Autodesk Inventor part; units mm, degrees
ref_plane "Work Plane1" through (0, 0, 0) normal (0, 0, 1) x (1, 0, 0)
ref_plane "Work Plane2" through (0, 0, 4) normal (0, 0, -1) x (-1, 0, 0)
ref_plane "Work Plane3" through (-20.3, -49, 28.5) normal (0, -1, 0) x (1, 0, 0)
ref_plane "Work Plane1" through (0, 0, 0) normal (0, 0, 1) x (1, 0, 0)
sketch "Sketch1" plane through (0, 0, 0) normal (0, 0, 1) x (1, 0, 0)
  circle A0 centre (-17.3, 4) radius 1.35
  circle A1 centre (-17.3, -18) radius 1.35
  circle A2 centre (-17.3, -40) radius 1.35
  line L0 (-17.3, 4) -> (-14.8, 4)
  line L1 (-14.8, 4) -> (-14.8, 9)
  line L2 (-14.8, 9) -> (-20.3, 9)
  line L3 (-17.3, -40) -> (-17.3, -54)
  line L4 (-14.8, 4) -> (-14.8, -54)
  line L5 (-14.8, -54) -> (-17.3, -54)
  line L6 (-17.3, -54) -> (-20.3, -54)
  line L7 (-20.3, -54) -> (-20.3, 9)
  point P0 (0, 0)
  dimension "d0" = 2.5
  dimension "d1" = 5
  dimension "d2" = 5.5
  dimension "d3" = 14
extrude "Extrusion1" add sketch "Sketch1" along normal blind 36.5
sketch "Sketch2" plane through (-20.3, -54, 0) normal (0, -1, 0) x (1, 0, 0)
  line L0 (0, 0) -> (5.5, 0)
  line L1 (5.5, 0) -> (5.5, 36.5)
  line L2 (0, 36.5) -> (5.5, 36.5)
  line L3 (0, 0) -> (0, 36.5)
  line L4 (2.75, 36.5) -> (2.75, 25.5)
  circle A0 centre (2.75, 25.5) radius 1.5
  point P0 (20.3, 0)
  dimension "d6" = 11
  dimension "d7" = 3
extrude "Extrusion2" cut sketch "Sketch2" against normal blind 10 contours A0
sketch "Sketch3" plane through (-20.3, -54, 0) normal (-1, 0, 0) x (0, 0, 1)
  line L0 (0, 63) -> (0, 0)
  line L1 (0, 0) -> (36.5, 0)
  line L2 (36.5, 63) -> (36.5, 0)
  line L3 (0, 63) -> (36.5, 63)
  line L4 (0, 0) -> (36.5, 0)
  line L5 (36.5, 0) -> (28.5, 0)
  line L6 (28.5, 0) -> (28.5, 8)
  line L7 (28.5, 8) -> (36.5, 8)
  line L8 (36.5, 8) -> (36.5, 0)
  point P0 (0, 54)
  dimension "d10" = 8
  dimension "d11" = 8
extrude "Extrusion3" cut sketch "Sketch3" against normal blind 10 contours L6 L7 L2 L1
sketch "Sketch4" plane through (-20.3, 9, 0) normal (0, 1, 0) x (1, 0, 0)
  line L0 (5.5, 0) -> (0, 0)
  line L1 (0, 0) -> (0, -36.5)
  line L2 (5.5, -36.5) -> (0, -36.5)
  line L3 (5.5, 0) -> (5.5, -36.5)
  line L4 (6.8, -6) -> (8.8, -6)
  line L5 (6.8, -6) -> (5.5, -6)
  line L6 (5.5, -6) -> (5.5, -6.5)
  line L7 (5.5, 0) -> (5.5, -28.5)
  line L8 (5.5, -6.5) -> (15.5, -6.5)
  line L9 (15.5, -6.5) -> (15.5, -11.5)
  line L10 (15.5, -11.5) -> (5.5, -11.5)
  line L11 (5.5, -11.5) -> (5.5, -6.5)
  point P0 (20.3, 0)
  dimension "d14" = 0.5
  dimension "d15" = 10
  dimension "d16" = 5
extrude "Extrusion4" add sketch "Sketch4" against normal up to surface (63 mm away) contours L8 L9 L10 L3
sketch "Sketch5" plane through (-4.8, 9, 6.5) normal (0, 0, -1) x (-1, 0, 0)
  circle A0 centre (12.5, -49) radius 1.35
  circle A1 centre (12.5, -27) radius 1.35
  circle A2 centre (12.5, -5) radius 1.35
  line L0 (10, -63) -> (10, 0)
  line L1 (15.5, -63) -> (10, -63)
  line L2 (15.5, 0) -> (15.5, -63)
  line L3 (10, 0) -> (15.5, 0)
  line L4 (0, -63) -> (10, -63)
  line L5 (10, 0) -> (10, -63)
  line L6 (0, 0) -> (10, 0)
  line L7 (0, 0) -> (0, -63)
  line L8 (-19.8, 5.5) -> (-16.3, 5.5)
  line L9 (-19.8, 5.5) -> (-24.9, -0.5)
  line L10 (-24.9, -0.5) -> (-24.9, -53.6)
  line L11 (-24.9, -53.6) -> (-19.8, -59.6)
  line L12 (-19.8, -59.6) -> (10.2, -59.6)
  line L13 (10.2, -59.6) -> (15.3, -53.6)
  line L14 (15.3, -53.6) -> (15.3, -0.5)
  line L15 (15.3, -0.5) -> (10.2, 5.5)
  line L16 (6.7, 5.5) -> (10.2, 5.5)
  arc A3 (9.7, 2.5) -> (6.7, 5.5) centre (6.7, 2.5) ccw
  line L17 (9.7, -51) -> (9.7, 2.5)
  arc A4 (6.7, -54) -> (9.7, -51) centre (6.7, -51) ccw
  line L18 (-16.3, -54) -> (6.7, -54)
  arc A5 (-19.3, -51) -> (-16.3, -54) centre (-16.3, -51) ccw
  line L19 (-19.3, 2.5) -> (-19.3, -51)
  arc A6 (-16.3, 5.5) -> (-19.3, 2.5) centre (-16.3, 2.5) ccw
  circle A7 centre (12.5, -5) radius 1.35
  circle A8 centre (12.5, -27) radius 1.35
  circle A9 centre (12.5, -49) radius 1.35
  circle A10 centre (6.2, -56.8) radius 1.35
  circle A11 centre (-22.1, -5) radius 1.35
  circle A12 centre (-22.1, -27) radius 1.35
  circle A13 centre (-22.1, -49) radius 1.35
  circle A14 centre (-15.8, -56.8) radius 1.35
  line L20 (10, 0) -> (10, -63)
  line L21 (10, -63) -> (0, -63)
  line L22 (0, -63) -> (0, -54.5)
  line L23 (0, -54.5) -> (10, -54.5)
  line L24 (10, -54.5) -> (10, -63)
  point P0 (-4.8, -9)
  dimension "d19" = 10
  dimension "d20" = 8.5
extrude "Extrusion5" add sketch "Sketch5" along normal up to surface (6.5 mm away) contours L0 L12 L7 L23 | L0 L4 L7 L12
ref_plane "Work Plane2" through (0, 0, 4) normal (0, 0, -1) x (-1, 0, 0)
sketch "Sketch6" plane through (0, 0, 4) normal (0, 0, -1) x (-1, 0, 0)
  circle A0 centre (17.3, 4) radius 1.35
  circle A1 centre (17.3, -18) radius 1.35
  circle A2 centre (11, -47.8) radius 1.35
  circle A3 centre (17.3, -40) radius 1.35
  circle A4 centre (17.3, -18) radius 1.35
  circle A5 centre (17.3, 4) radius 1.35
  line L0 (20.3, -54) -> (4.8, -54)
  line L1 (20.3, 9) -> (20.3, -54)
  line L2 (14.8, 9) -> (20.3, 9)
  line L3 (14.8, -45.5) -> (14.8, 9)
  line L4 (14.8, -45.5) -> (4.8, -45.5)
  line L5 (4.8, -45.5) -> (4.8, -54)
  circle A6 centre (11, -47.8) radius 1.35
  circle A7 centre (11, -47.8) radius 1.35
  line L6 (17.3, 4) -> (17.3, 6.6)
  line L7 (18.8011, 6.6) -> (20.3022, 4)
  line L8 (20.3022, 4) -> (18.8011, 1.4)
  line L9 (18.8011, 1.4) -> (15.7989, 1.4)
  line L10 (15.7989, 1.4) -> (14.2978, 4)
  line L11 (14.2978, 4) -> (15.7989, 6.6)
  line L12 (15.7989, 6.6) -> (18.8011, 6.6)
  line L13 (18.8011, 1.4) -> (28.5961, 1.4)
  line L14 (28.5961, 1.4) -> (28.5961, 6.6)
  line L15 (28.5961, 6.6) -> (18.8011, 6.6)
  line L16 (18.8011, 6.6) -> (18.8011, 1.4)
  line L17 (11, -47.8) -> (13.6, -47.8)
  line L18 (13.6, -49.3011) -> (11, -50.8022)
  line L19 (11, -50.8022) -> (8.4, -49.3011)
  line L20 (8.4, -49.3011) -> (8.4, -46.2989)
  line L21 (8.4, -46.2989) -> (11, -44.7978)
  line L22 (11, -44.7978) -> (13.6, -46.2989)
  line L23 (13.6, -46.2989) -> (13.6, -49.3011)
  line L24 (13.6, -49.3011) -> (8.4, -49.3011)
  line L25 (8.4, -49.3011) -> (8.4, -56.2377)
  line L26 (8.4, -56.2377) -> (13.6, -56.2377)
  line L27 (13.6, -56.2377) -> (13.6, -49.3011)
  line L28 (18.8011, -15.4) -> (20.3022, -18)
  line L29 (20.3022, -18) -> (18.8011, -20.6)
  line L30 (18.8011, -20.6) -> (28.5961, -20.6)
  line L31 (28.5961, -20.6) -> (28.5961, -15.4)
  line L32 (28.5961, -15.4) -> (18.8011, -15.4)
  line L33 (18.8011, -15.4) -> (18.8011, -20.6)
  line L34 (17.3, -18) -> (17.3, -15.4)
  line L35 (18.8011, -20.6) -> (15.7989, -20.6)
  line L36 (15.7989, -15.4) -> (18.8011, -15.4)
  line L37 (15.7989, -20.6) -> (14.2978, -18)
  line L38 (14.2978, -18) -> (15.7989, -15.4)
  line L39 (18.8011, -37.4) -> (20.3022, -40)
  line L40 (20.3022, -40) -> (18.8011, -42.6)
  line L41 (18.8011, -42.6) -> (28.5961, -42.6)
  line L42 (28.5961, -42.6) -> (28.5961, -37.4)
  line L43 (28.5961, -37.4) -> (18.8011, -37.4)
  line L44 (18.8011, -37.4) -> (18.8011, -42.6)
  line L45 (17.3, -40) -> (17.3, -37.4)
  line L46 (18.8011, -42.6) -> (15.7989, -42.6)
  line L47 (15.7989, -37.4) -> (18.8011, -37.4)
  line L48 (15.7989, -42.6) -> (14.2978, -40)
  line L49 (14.2978, -40) -> (15.7989, -37.4)
  point P0 (0, 0)
  dimension "d24" = 2.6
  dimension "d25" = 2.6
  dimension "d28" = 22
extrude "Extrusion6" cut sketch "Sketch6" against normal blind 3 contours L12 L16 L9 L10 L3 L11 | L15 L1 L7 | L7 L8 L16 | L3 L10 L11 | L1 L15 L14 L13 | L1 L13 L8 | L38 L36 L33 L35 L37 L3 | L3 L37 L38 | L32 L31 L30 L1 | L1 L28 L32 | L29 L33 L28 | L1 L30 L29 | L49 L47 L44 L46 L48 L3 | L3 L48 L49 | L43 L42 L41 L1 | L1 L39 L43 | L40 L44 L39 | L1 L41 L40 | A2 | L22 L23 L24 L20 L21 L4 | L4 L21 L22 | L27 L26 L25 L0 | L0 L25 L19 L18 L27 | L24 L18 L19
sketch "Sketch7" plane through (0, 0, 36.5) normal (0, 0, 1) x (1, 0, 0)
  line L0 (-20.3, -46) -> (-14.8, -46)
  line L1 (-14.8, -46) -> (-14.8, 9)
  line L2 (-14.8, 9) -> (-20.3, 9)
  line L3 (-20.3, 9) -> (-20.3, -46)
  circle A0 centre (-17.3, 4) radius 1.35
  circle A1 centre (-17.3, -18) radius 1.35
  circle A2 centre (-17.3, -40) radius 1.35
  point P0 (0, 0)
extrude "Extrusion7" add sketch "Sketch7" against normal blind 25 contours A0 | A1 | A2
ref_plane "Work Plane3" through (-20.3, -49, 28.5) normal (0, -1, 0) x (1, 0, 0)
sketch "Sketch8" plane through (-20.3, -49, 28.5) normal (0, -1, 0) x (1, 0, 0)
  circle A0 centre (2.75, -3) radius 1.5
  line L0 (2.75, -3) -> (2.75, -0.4)
  line L1 (4.2511, -0.4) -> (5.7522, -3)
  line L2 (5.7522, -3) -> (4.2511, -5.6)
  line L3 (4.2511, -5.6) -> (1.2489, -5.6)
  line L4 (1.2489, -5.6) -> (-0.2522, -3)
  line L5 (-0.2522, -3) -> (1.2489, -0.4)
  line L6 (1.2489, -0.4) -> (4.2511, -0.4)
  line L7 (1.2489, -0.4) -> (-2.7612, -0.4)
  line L8 (-2.7612, -0.4) -> (-2.7612, -5.6)
  line L9 (-2.7612, -5.6) -> (1.2489, -5.6)
  line L10 (1.2489, -5.6) -> (1.2489, -0.4)
  point P0 (20.3, -28.5)
  dimension "d38" = 2.6
extrude "Extrusion8" cut sketch "Sketch8" against normal blind 3 contours A0 L0 L6 L1 L2 L3 L10 | A0 L10 L6 L0 | L10 L4 L5 | L9 L8 L7 L5 L4
sketch "Sketch9" plane through (-20.3, 9, 0) normal (0, 1, 0) x (1, 0, 0)
  line L0 (5.5, 0) -> (0, 0)
  line L1 (0, 0) -> (0, -36.5)
  line L2 (5.5, -36.5) -> (0, -36.5)
  line L3 (5.5, -11.5) -> (5.5, -36.5)
  line L4 (5.5, -11.5) -> (15.5, -11.5)
  line L5 (15.5, -11.5) -> (15.5, -6.5)
  line L6 (15.5, -6.5) -> (5.5, -6.5)
  line L7 (5.5, 0) -> (5.5, -6.5)
  line L8 (5.5, -11.5) -> (15.5, -11.5)
  line L9 (5.5, -11.5) -> (5.5, -28.5)
  line L10 (15.5, -11.5) -> (5.5, -11.5)
  line L11 (5.5, -20) -> (15.5, -20)
  line L12 (5.5, -20) -> (11.5, -20)
  line L13 (5.5, -24) -> (5.5, -20)
  line L14 (15.5, -24) -> (15.5, -27)
  line L15 (15.5, -27) -> (5.5, -27)
  line L16 (5.5, -27) -> (5.5, -24)
  line L17 (5.5, -11.5) -> (15.5, -11.5)
  line L18 (15.5, -11.5) -> (15.5, -16)
  line L19 (15.5, -16) -> (5.5, -16)
  line L20 (5.5, -16) -> (5.5, -11.5)
  line L21 (5.5, -16) -> (11.5, -16)
  line L22 (11.5, -16) -> (11.5, -20)
  line L23 (11.5, -20) -> (5.5, -20)
  line L24 (5.5, -20) -> (5.5, -16)
  line L25 (5.5, -20) -> (15.5, -20)
  line L26 (15.5, -20) -> (15.5, -27)
  line L27 (15.5, -27) -> (5.5, -27)
  line L28 (5.5, -27) -> (5.5, -20)
  point P0 (20.3, 0)
  dimension "d41" = 8.5
  dimension "d44" = 10
  dimension "d45" = 3
  dimension "d48" = 4.5
extrude "Extrusion9" add sketch "Sketch9" against normal up to surface (63 mm away) contours L18 L19 L3 L4 | L3 L11 L26 L14 L15 | L19 L22 L11 L3
sketch "Sketch10" plane through (-20.3, -54, 28.5) normal (0, -1, 0) x (1, 0, 0)
  point P0 (20.3, -28.5)
sketch "Sketch11" plane through (-20.3, -54, 28.5) normal (0, 0, 1) x (1, 0, 0)
  line L0 (5.5, 8) -> (5.5, 0)
  line L1 (0, 8) -> (5.5, 8)
  line L2 (0, 0) -> (0, 8)
  line L3 (5.5, 0) -> (0, 0)
  point P0 (20.3, 54)
extrude "Extrusion10" add sketch "Sketch11" along normal blind 2
properties part number "side"
Geometry check sheet. Reference: the model listing, model coordinates, mm. A direction names the side the tool comes from. Round coordinates to 2 decimals unless told otherwise and drop trailing zeros. Write each loop counter-clockwise with the first axis right and the second up, starting at its lowest first coordinate (ties: lowest second). Pieces come first, ordered by that corner, then holes. Notation, with made-up numbers: (-25, 39) - (18, 39) arc R11 ccw to (18, 58) - close; hole circle Ø1 at (-29.5, 8.5). An arc over 180 degrees is marked (long way). Write each question's results on one line, items separated by ' | '.
(1) Draft check along X on faces 6 (the face through (-16.8, -45, 26.8)), 7 (the face through (-4.8, -22, 23)), 8 (the face through (-10, -22, 27)), 9 (the face through (-15.205, -16.429, 5.479)). Enter one of: pulls with the +X half, pulls with the -X half, needs draft (parallel to the pull), parting line crosses it, or undercut.
Computed:
face 6: undercut | face 7: pulls with the +X half | face 8: needs draft | face 9: pulls with the -X half
(2) Sectioned sample at A-A, the plane z = 8. Enter the section's corners in (x, y).
Computed:
outline: (-20.3, -54) - (-4.8, -54) - (-4.8, 9) - (-20.3, 9) - close; hole circle Ø2.7 at (-17.3, -40); hole circle Ø2.7 at (-17.3, -18); hole circle Ø2.7 at (-17.3, 4)
(3) Set-up check for faces 1 (the face through (-14.8, -22, 32)), 2 (the face through (-17, -18, 11.5)), 3 (the face through (-19, -17, 7)), 4 (the face through (-12.86, -45.87, 5.48)), 5 (the face through (-7, -22, 20)): record each of +Z, -Z, +X, -X, +Y, -Y from which the full face is reachable in a straight line by a thin tool's end or side.
Computed:
face 1: +Z, +X, +Y, -Y | face 2: -Z | face 3: -X | face 4: -Y | face 5: +X, +Y, -Y
(4) Sectioned sample at C-C, the plane z = 29.5. Enter the section's corners in (x, y), plus the area to 4 significant figures.
Computed:
outline: (-20.3, -54) - (-14.8, -54) - (-14.8, 9) - (-20.3, 9) - close | area: 346.5 mm^2
(5) Sectioned sample at B-B, the plane y = -47.8. Enter the section's corners in (x, z).
Computed:
outline: (-20.3, 0) - (-12.35, 0) - (-12.35, 4) - (-13.6, 4) - (-13.6, 7) - (-8.4, 7) - (-8.4, 4) - (-9.65, 4) - (-9.65, 0) - (-4.8, 0) - (-4.8, 16) - (-8.8, 16) - (-8.8, 20) - (-4.8, 20) - (-4.8, 27) - (-14.8, 27) - (-14.8, 30.5) - (-20.3, 30.5) - (-20.3, 28.1) - (-16.05, 28.1) - (-14.8, 25.94) - (-14.8, 25.06) - (-16.05, 22.9) - (-20.3, 22.9) - close
(6) Thickness scan on probe 1 along Y at (x, z) = (-17.3, 10.2); probe 2 along X at (y, z) = (-18, 3); probe 3 along Z at (x, y) = (-8, -3.5). Record the ranges inside material, lowest first. Write a range as from..to.
Computed:
probe 1: y = -54..-41.35, -38.65..-19.35, -16.65..2.65, 5.35..9 | probe 2: x = -20.3..-18.65, -15.95..-14.8 | probe 3: z = 6.5..16, 20..27
(7) Depth check by flat-ended pin: pin 1 Ø0.9 at (x, y) = (-18.5, -48) entering from -Z; pin 2 Ø4.5 at (x, y) = (-7.5, -36.5) entering from +Z; pin 3 Ø1 at (x, y) = (-12, -33) entering from -Z; pin 4 Ø3 at (y, z) = (-34, 33) entering from +X. Enter the tip coordinate at first touch or a pass-through.
Computed:
pin 1: stops at z = 0 | pin 2: stops at z = 27 | pin 3: stops at z = 6.5 | pin 4: stops at x = -14.8
(8) Sectioned sample at D-D, the plane y = -21.5. Enter the section's corners in (x, z).
Computed:
outline: (-20.3, 0) - (-14.8, 0) - (-14.8, 6.5) - (-4.8, 6.5) - (-4.8, 16) - (-8.8, 16) - (-8.8, 20) - (-4.8, 20) - (-4.8, 27) - (-14.8, 27) - (-14.8, 36.5) - (-20.3, 36.5) - close
